Verification items for the finished model (mm, model axes). A direction names the side the tool comes from. Coordinates: 2 decimals unless noted, no trailing zeros. Loops run counter-clockwise (first coordinate to the right, second up) from the corner with the lowest first, then second, coordinate; pieces in that order, holes last. Notation, with made-up numbers: (28.5, 13) - (41.5, 13) arc R11 cw to (41.5, 27) - close; hole circle Ø1 at (-10.75, -8). An arc over 180 degrees is marked (long way). Answer as CSV lines item,"result". Start each with the question number.
1. Gauge pin test, flat ends, axial feed: P1, Ø3, axis at x = 31.5, z = 38, coming from the -Y side; P2, Ø3, axis at y = 32.5, z = -20.5, coming from the -X side; P3, Ø4.5, axis at x = -22.5, z = 9.5, coming from the +Y side; P4, Ø1.6, axis at x = -51.5, z = 45.5, coming from the -Y side. Record the tip position at first contact, or that the pin passes through.
2. Cross-section at C-C (z = -31). Enter the section's corners in (x, y).
3. Release check for a two-part mould opening along Y. For faces 4 (the flat face through (-50, 47, 35)), 5 (the cylindrical face through (-50.4, 47.1, 12.5)), 6 (the flat face through (-1, 0, -1)), 7 (the flat face through (-52, 25, 15)) record: pulls with the +Y half, pulls with the -Y half, needs draft (parallel to the pull), parting line crosses it, or undercut.
4. Material ranges on line 1 (Y direction, x = -50.4, z = 15); line 2 (Y direction, x = -50.2, z = 35); line 3 (X direction, y = 54, z = 17), recorded low to high. Write a range as [from, to].
5. Cross-section at A-A (x = -22.5). Enter the section's corners in (y, z), plus the area to 3 significant figures.
6. Set-up check for faces 1 (the cylindrical face through (-50.37, 43.621, 38.685)), 2 (the flat face through (-14.65, 55.94, 33.13)), 3 (the flat face through (-34, 60, 28)): record each of +Z, -Z, +X, -X, +Y, -Y from which the full face is reachable in a straight line by a thin tool's end or side.
```python
from build123d import *
from build123d.topology import SkipClean

# Parameters (mm, degrees)
SKETCH_1_W          = 100
SKETCH_1_H          = 100
EXTRUDE_1_DEPTH     = 60
SKETCH_2_W          = 45
SKETCH_2_H          = 45
CUT_EXTRUDE_1_DEPTH = 8
SKETCH_3_W          = 10
SKETCH_3_H          = 20
EXTRUDE_2_DEPTH     = 2
SKETCH_4_W          = 20
SKETCH_4_H          = 10
SKETCH_4_W_2        = 10
EXTRUDE_3_DEPTH     = 2
SKETCH_5_R          = 5
SKETCH_5_R_2        = 2.5
EXTRUDE_4_DEPTH     = 2
FILLET_1_R          = 1.25
FILLET_2_R          = 1.25
EXTRUDE_5_DEPTH     = 8
SKETCH_7_R          = 5
EXTRUDE_6_DEPTH     = 2


with BuildPart() as part:
    # 草图1 → 凸台-拉伸1 (new body)
    with BuildSketch(Plane(origin=(0, 0, 0), x_dir=(1, 0, 0), z_dir=(0, 1, 0))):
        Rectangle(SKETCH_1_W, SKETCH_1_H)
    extrude(amount=EXTRUDE_1_DEPTH)

    # 草图2 → 切除-拉伸1 (cut)
    with BuildSketch(Plane(origin=(0, 60, 0), x_dir=(1, 0, 0), z_dir=(0, 1, 0))):
        with Locations((-22.5, -22.5)):
            Rectangle(SKETCH_2_W, SKETCH_2_H)
    extrude(amount=-CUT_EXTRUDE_1_DEPTH, mode=Mode.SUBTRACT)

    # 草图3 → 凸台-拉伸2 (add)
    with BuildSketch(Plane(origin=(0, 60, 0), x_dir=(1, 0, 0), z_dir=(0, 1, 0))):
        with Locations((-38, 30)):
            Rectangle(SKETCH_3_W, SKETCH_3_H)
        with Locations((-20, 30)):
            Rectangle(SKETCH_3_W, SKETCH_3_H)
    extrude(amount=EXTRUDE_2_DEPTH)

    # 草图4 → 凸台-拉伸3 (add)
    with BuildSketch(Plane.ZY.offset(50)):
        with Locations((15, 25)):
            Rectangle(SKETCH_4_W, SKETCH_4_H)
        with Locations((44, 30)):
            Rectangle(SKETCH_4_W_2, SKETCH_4_H)
    extrude(amount=EXTRUDE_3_DEPTH)

    # 草图5 → 凸台-拉伸4 (add)
    # profile 1 of 2: a face of its own
    with BuildSketch(Plane.ZY.offset(50)):
        with Locations(Location((15, 47, 0), (0, 0, 180))):
            Circle(SKETCH_5_R)
        with Locations((15, 47)):
            Circle(SKETCH_5_R_2, mode=Mode.SUBTRACT)
    # profile 2 of 2: a face of its own
    with BuildSketch(Plane.ZY.offset(50)):
        with Locations(Location((35, 47, 0), (0, 0, 180))):
            Circle(SKETCH_5_R)
        with Locations((35, 47)):
            Circle(SKETCH_5_R_2, mode=Mode.SUBTRACT)
    extrude(amount=EXTRUDE_4_DEPTH)

    # 圆角1
    fillet_1_edges = [part.edges().sort_by_distance(p)[0] for p in [
        (-52, 47, 20),
        (-52, 47, 12.5),
    ]]
    fillet(fillet_1_edges, radius=FILLET_1_R - 0.0001)  # a hair under: the kernel refuses the full size

    # 圆角2
    fillet_2_edges = [part.edges().sort_by_distance(p)[0] for p in [
        (-52, 47, 40),
        (-52, 47, 32.5),
    ]]
    fillet(fillet_2_edges, radius=FILLET_2_R - 0.0001)  # a hair under: the kernel refuses the full size

    # 草图6 → 凸台-拉伸5 (add)
    with BuildSketch(Plane(origin=(0, 52, 0), x_dir=(1, 0, 0), z_dir=(0, 1, 0))):
        with BuildLine():
            Line((-25.5, -18.5), (-30, -2.5))
            Line((-30, -2.5), (-15, -2.5))
            Line((-15, -2.5), (-19.5, -18.5))
            ThreePointArc((-19.5, -18.5), (-18.169872981, -20), (-17.535898385, -21.901923789))
            Line((-17.535898385, -21.901923789), (-1.429491924, -26.004809472))
            Line((-1.429491924, -26.004809472), (-8.929491924, -38.995190528))
            Line((-8.929491924, -38.995190528), (-20.535898385, -27.098076211))
            ThreePointArc((-20.535898385, -27.098076211), (-22.5, -27.5), (-24.464101615, -27.098076211))
            Line((-24.464101615, -27.098076211), (-36.070508076, -38.995190528))
            Line((-36.070508076, -38.995190528), (-43.570508076, -26.004809472))
            Line((-43.570508076, -26.004809472), (-27.464101615, -21.901923789))
            ThreePointArc((-27.464101615, -21.901923789), (-26.830127019, -20), (-25.5, -18.5))
        make_face()
    extrude(amount=EXTRUDE_5_DEPTH)

    # 草图7 → 凸台-拉伸6 (add)
    with SkipClean():  # the faces are left unmerged after this step: merging them gives an invalid solid
        with BuildSketch(Plane(origin=(0, 60, 0), x_dir=(1, 0, 0), z_dir=(0, 1, 0))):
            with Locations(Location((-22.5, -22.5, 0), (0, 0, 53.130102354))):
                Circle(SKETCH_7_R)
        extrude(amount=EXTRUDE_6_DEPTH)


solid = part.part
```
Values follow:
1,P1,"stops at y = 0"
1,P2,"stops at x = -50"
1,P3,"stops at y = 60"
1,P4,"stops at y = 25"
2,outline,"(-50, 0) - (50, 0) - (50, 60) - (-15, 60) - (-15, 62) - (-25, 62) - (-25, 60) - (-33, 60) - (-33, 62) - (-43, 62) - (-43, 60) - (-50, 60) - close"
3,face 4,"undercut"
3,face 5,"undercut"
3,face 6,"pulls with the -Y half"
3,face 7,"needs draft"
4,line 1,"y = [20, 30], [42, 44.5], [49.5, 52]"
4,line 2,"y = [42, 44.5], [49.5, 52]"
4,line 3,"x = [-50, -45], [-25.92, -19.08], [0, 50]"
5,outline,"(0, -50) - (60, -50) - (60, -40) - (62, -40) - (62, -20) - (60, -20) - (60, 0) - (52, 0) - (52, 2.5) - (60, 2.5) - (60, 17.5) - (62, 17.5) - (62, 27.5) - (52, 27.5) - (52, 45) - (60, 45) - (60, 50) - (0, 50) - close"
5,area,"5,900 mm²"
6,face 1,"-X"
6,face 2,"+Y"
6,face 3,"+Z, -X, +Y"
